```python
from build123d import *

# Parameters (mm, degrees)
F0_R          = 28.619022
F1_DEPTH      = 95.800422
F2_W          = 90.508705
F2_H          = 21.804128
F3_DEPTH      = 93.832932
F3_DEPTH_BACK = 25.4


with BuildPart() as f1:
    # F0 (on Top) → F1 (new body)
    with BuildSketch(Plane.XY):
        with Locations((24.492977, -28.250135)):
            Circle(F0_R)
    extrude(amount=F1_DEPTH)

    # F2 (on Front) → F3 (join, two sides)
    with BuildSketch(Plane.XZ) as f3_sk:
        with Locations((21.254842, 21.079259)):
            Rectangle(F2_W, F2_H)
    extrude(amount=F3_DEPTH)
    extrude(f3_sk.sketch, amount=-F3_DEPTH_BACK)


solid = f1.part
```
Check sheet for the modelled part. Datum: model origin and axes. Units: mm. A direction names the side the tool comes from. Round coordinates to 2 decimals unless told otherwise and drop trailing zeros. Order: outer loops, then holes, each group sorted by start corner. A loop starts at its lowest first (then second) coordinate and runs counter-clockwise, first axis right, second up.
1) Section check B-B (y = -35). Record the boundary of the cut face in (x, z), and give its area (3 significant figures).
2) Section check D-D (z = 88.5). Record the boundary of the cut face in (x, y).
3) Section check A-A (x = 47). Record the boundary of the cut face in (y, z).
4) Section check C-C (y = -59). Record the boundary of the cut face in (x, z), and give its area (3 significant figures).
5) Go/stop test with flat-tipped pins: pin 1 Ø5 at (x, z) = (14, 84.5) entering from -Y; pin 2 Ø6 at (y, z) = (-52, 79.5) entering from +X; pin 3 Ø1 at (y, z) = (-47, 54.5) entering from +X. Record where each tip stops, or that it passes through.
6) Scan lines: line 1 (Z direction, x = -20, y = -6.5); line 2 (Y direction, x = 25.5, z = 89); line 3 (X direction, y = -27, z = 38). Record each from-to range of solid material in increasing order.
7) Tool access check on faces 1 (the cylindrical face through (51.79, -19.65, 63.44)), 2 (the cylindrical face through (51.79, -19.65, 5.02)), 3 (the flat face through (66.509, -35, 21)). Record the directions out of +Z, -Z, +X, -X, +Y, -Y that give a thin tool (end or side, any length) a straight path to the whole face; none if there is none.
Result:
1. outline: (-24, 10.18) - (-3.32, 10.18) - (-3.32, 0) - (52.3, 0) - (52.3, 10.18) - (66.51, 10.18) - (66.51, 31.98) - (52.3, 31.98) - (52.3, 95.8) - (-3.32, 95.8) - (-3.32, 31.98) - (-24, 31.98) - close
1. area: 6,090 mm2
2. outline: circle Ø57.24 at (24.49, -28.25)
3. outline: (-93.83, 10.18) - (-45.93, 10.18) - (-45.93, 0) - (-10.57, 0) - (-10.57, 10.18) - (25.4, 10.18) - (25.4, 31.98) - (-10.57, 31.98) - (-10.57, 95.8) - (-45.93, 95.8) - (-45.93, 31.98) - (-93.83, 31.98) - close
4. outline: (-24, 10.18) - (66.51, 10.18) - (66.51, 31.98) - (-24, 31.98) - close
4. area: 1,970 mm2
5. pin 1: stops at y = -55.73
5. pin 2: stops at x = 44.2
5. pin 3: stops at x = 46.54
6. line 1: z = 10.18 to 31.98
6. line 2: y = -56.85 to 0.35
6. line 3: x = -4.1 to 53.08
7. face 1: +Z
7. face 2: -Z
7. face 3: +Z, -Z, +X, +Y, -Y
